from build123d import *

# Parameters (mm, degrees)
SKETCH1_R               = 12.5
BOSS_EXTRUDE1_DEPTH     = 40
SKETCH6_W               = 5
SKETCH6_H               = 25
BOSS_EXTRUDE3_DEPTH     = 6.5
BOSS_EXTRUDE4_DEPTH     = 5
CUT_EXTRUDE1_DEPTH      = 45.511234537
CUT_EXTRUDE1_DEPTH_BACK = 45.511234537
SKETCH10_R              = 2.5
SKETCH12_W              = 4.8936145
SKETCH12_H              = 25
CUT_EXTRUDE2_DEPTH      = 17.5
CUT_EXTRUDE3_DEPTH      = 44.732139211
CUT_EXTRUDE3_DEPTH_BACK = 44.732139211
SKETCH13_R              = 2.5


with BuildPart() as part:
    # Sketch1 → Boss-Extrude1 (new body)
    with BuildSketch(Plane(origin=(0, 0, 0), x_dir=(0, 0, -1), z_dir=(1, 0, 0))):
        Circle(SKETCH1_R)
    extrude(amount=-BOSS_EXTRUDE1_DEPTH)

    # Sketch6 → Boss-Extrude3 (add)
    with BuildSketch(Plane(origin=(0, 0, 0), x_dir=(0, 0, -1), z_dir=(1, 0, 0))):
        Rectangle(SKETCH6_W, SKETCH6_H)
    extrude(amount=BOSS_EXTRUDE3_DEPTH)

    # Sketch8 → Boss-Extrude4 (add)
    with BuildSketch(Plane.XY.offset(2.5)):
        with BuildLine():
            Line((6.5, 12.5), (6.5, -12.5))
            ThreePointArc((6.5, -12.5), (19, 0), (6.5, 12.5))
        make_face()
    extrude(amount=-BOSS_EXTRUDE4_DEPTH)

    # Sketch10 → Cut-Extrude1 (cut, two sides: drawn at the far end of the back side and taken through both)
    with BuildSketch(Plane.XY.offset(2.5).offset(-CUT_EXTRUDE1_DEPTH_BACK)):
        with Locations((15.9, 0)):
            Circle(SKETCH10_R)
    extrude(amount=CUT_EXTRUDE1_DEPTH + CUT_EXTRUDE1_DEPTH_BACK, mode=Mode.SUBTRACT)

    # Sketch12 → Cut-Extrude2 (cut)
    with BuildSketch(Plane.ZY.offset(40)):
        Rectangle(SKETCH12_W, SKETCH12_H)
    extrude(amount=-CUT_EXTRUDE2_DEPTH, mode=Mode.SUBTRACT)

    # Sketch13 → Cut-Extrude3 (cut, two sides: drawn at the far end of the back side and taken through both)
    with BuildSketch(Plane.XY.offset(-CUT_EXTRUDE3_DEPTH_BACK)):
        with Locations((-35, 0)):
            Circle(SKETCH13_R)
    extrude(amount=CUT_EXTRUDE3_DEPTH + CUT_EXTRUDE3_DEPTH_BACK, mode=Mode.SUBTRACT)


solid = part.part
Geometry check sheet. Reference: the model listing, model coordinates, mm. A direction names the side the tool comes from. Round coordinates to 2 decimals unless told otherwise and drop trailing zeros. Loops run counter-clockwise (first coordinate to the right, second up) from the corner with the lowest first, then second, coordinate; pieces in that order, holes last. Notation, with made-up numbers: (31.5, 57.5) - (89.5, 57.5) arc R19 cw to (89.5, 78.5) - close; hole circle Ø5 at (-39.5, -19.5). An arc over 180 degrees is marked (long way). Answer as CSV lines item,"result".
(1) Cross-section at D-D, the plane z = 9.25. Enter the section's corners in (x, y), and give its area (3 significant figures).
Output values:
outline,"(-40, -8.41) - (0, -8.41) - (0, 8.41) - (-40, 8.41) - close; hole circle Ø5 at (-35, 0)"
area,"653 mm²"
(2) Material ranges on line 1 along X through (y, z) = (0, 8.25); line 2 along X through (y, z) = (0, 1.1); line 3 along Z through (x, y) = (-8.5, -2.5), recorded low to high.
Output values:
line 1,"x = -40 to -37.5, -32.5 to 0"
line 2,"x = -22.5 to 13.4, 18.4 to 19"
line 3,"z = -12.25 to 12.25"
(3) Cross-section at C-C, the plane x = 15.9. Enter the section's corners in (y, z), and give its area (3 significant figures).
Output values:
outline,"(-8.24, -2.5) - (-2.5, -2.5) - (-2.5, 2.5) - (-8.24, 2.5) - close; (2.5, -2.5) - (8.24, -2.5) - (8.24, 2.5) - (2.5, 2.5) - close"
area,"57.4 mm²"
(4) Set-up check for faces 1 (the face through (-31, 0, -2.447)), 2 (the face through (0, 0, -6)), 3 (the face through (7, 0, 2.5)): record each of +Z, -Z, +X, -X, +Y, -Y from which the full face is reachable in a straight line by a thin tool's end or side.
Output values:
face 1,"-X, +Y, -Y"
face 2,"-Z, +X, +Y, -Y"
face 3,"+Z, +X, +Y, -Y"
(5) Cross-section at B-B, the plane y = 0. Enter the section's corners in (x, z).
Output values:
outline,"(-40, -12.5) - (-37.5, -12.5) - (-37.5, -2.45) - (-40, -2.45) - close; (-40, 2.45) - (-37.5, 2.45) - (-37.5, 12.5) - (-40, 12.5) - close; (-32.5, -12.5) - (0, -12.5) - (0, -2.5) - (13.4, -2.5) - (13.4, 2.5) - (0, 2.5) - (0, 12.5) - (-32.5, 12.5) - (-32.5, 2.45) - (-22.5, 2.45) - (-22.5, -2.45) - (-32.5, -2.45) - close; (18.4, -2.5) - (19, -2.5) - (19, 2.5) - (18.4, 2.5) - close"
(6) Cross-section at A-A, the plane x = -35. Enter the section's corners in (y, z), and give its area (3 significant figures).
Output values:
outline,"(-12.26, -2.45) arc R12.5 ccw to (-2.5, -12.25) - (-2.5, -2.45) - close; (-12.26, 2.45) - (-2.5, 2.45) - (-2.5, 12.25) arc R12.5 ccw to start; (2.5, -12.25) arc R12.5 ccw to (12.26, -2.45) - (2.5, -2.45) - close; (2.5, 2.45) - (12.26, 2.45) arc R12.5 ccw to (2.5, 12.25) - close"
area,"270 mm²"
(7) Depth check by flat-ended pin: pin 1 Ø2 at (x, z) = (-24.5, -5) entering from +Y; pin 2 Ø5.5 at (x, y) = (13.5, -2.5) entering from -Z; pin 3 Ø1.5 at (x, z) = (-0.5, -8.5) entering from +Y. Enter the tip coordinate at first touch or a pass-through.
Output values:
pin 1,"stops at y = 11.84"
pin 2,"stops at z = -2.5"
pin 3,"stops at y = 9.81"
(8) Release check for a two-part mould opening along X. For faces 4 (the face through (18.285, 0.751, -0.035)), 5 (the face through (3, 12.5, 0)), 6 (the face through (-22.5, 0, 0)), 7 (the face through (0, 0, 6)) record: released by +X, released by -X, zero draft, split by the parting line, or undercut.
Output values:
face 4,"undercut"
face 5,"zero draft"
face 6,"released by -X"
face 7,"released by +X"
